Check sheet for the modelled part. Datum: model origin and axes. Units: mm. Coordinates: 2 decimals unless noted, no trailing zeros. Loops run counter-clockwise (first coordinate to the right, second up) from the corner with the lowest first, then second, coordinate; pieces in that order, holes last.
from build123d import *

# Parameters (mm, degrees)
SKETCH1_R           = 1.5
BOSS_EXTRUDE1_DEPTH = 5
SKETCH8_R           = 1.5
CUT_EXTRUDE5_DEPTH  = 10
SKETCH9_R           = 1.5
CUT_EXTRUDE6_DEPTH  = 10


with BuildPart() as part:
    # Sketch1 → Boss-Extrude1 (new body)
    with BuildSketch(Plane(origin=(0, 0, 0), x_dir=(1, 0, 0), z_dir=(0, 1, 0))):
        with BuildLine():
            Line((100, -40), (100, 10))
            Line((100, 10), (40, 150))
            Line((40, 150), (-40, 150))
            Line((-40, 150), (-100, 10))
            Line((-100, 10), (-100, -40))
            ThreePointArc((-100, -40), (-97.071067812, -47.071067812), (-90, -50))
            Line((-90, -50), (-70, -50))
            Line((-70, -50), (-70, -60))
            Line((-70, -60), (-70, -110))
            ThreePointArc((-70, -110), (-67.071067812, -117.071067812), (-60, -120))
            Line((-60, -120), (60, -120))
            ThreePointArc((60, -120), (67.071067812, -117.071067812), (70, -110))
            Line((70, -110), (70, -60))
            Line((70, -60), (70, -50))
            Line((70, -50), (90, -50))
            ThreePointArc((90, -50), (97.071067812, -47.071067812), (100, -40))
        make_face()
        with Locations((-60, -60)):
            Circle(SKETCH1_R, mode=Mode.SUBTRACT)
        with Locations((60, -60)):
            Circle(SKETCH1_R, mode=Mode.SUBTRACT)
    extrude(amount=BOSS_EXTRUDE1_DEPTH)

    # Sketch8 → Cut-Extrude5 (cut)
    with BuildSketch(Plane(origin=(0, 5, 0), x_dir=(1, 0, 0), z_dir=(0, 1, 0))):
        with Locations((-90, 10)):
            Circle(SKETCH8_R)
        with Locations((-32, 140)):
            Circle(SKETCH8_R)
        with Locations((90, 10)):
            Circle(SKETCH8_R)
        with Locations((32, 140)):
            Circle(SKETCH8_R)
    extrude(amount=-CUT_EXTRUDE5_DEPTH, mode=Mode.SUBTRACT)

    # Sketch9 → Cut-Extrude6 (cut)
    with BuildSketch(Plane(origin=(0, 5, 0), x_dir=(1, 0, 0), z_dir=(0, 1, 0))):
        with Locations((47.5, -50)):
            Circle(SKETCH9_R)
        with Locations((32.5, -50)):
            Circle(SKETCH9_R)
        with Locations((32.5, -92)):
            Circle(SKETCH9_R)
        with Locations((-32.5, -50)):
            Circle(SKETCH9_R)
        with Locations((-32.5, -92)):
            Circle(SKETCH9_R)
        with Locations((-47.5, -50)):
            Circle(SKETCH9_R)
    extrude(amount=-CUT_EXTRUDE6_DEPTH, mode=Mode.SUBTRACT)


solid = part.part
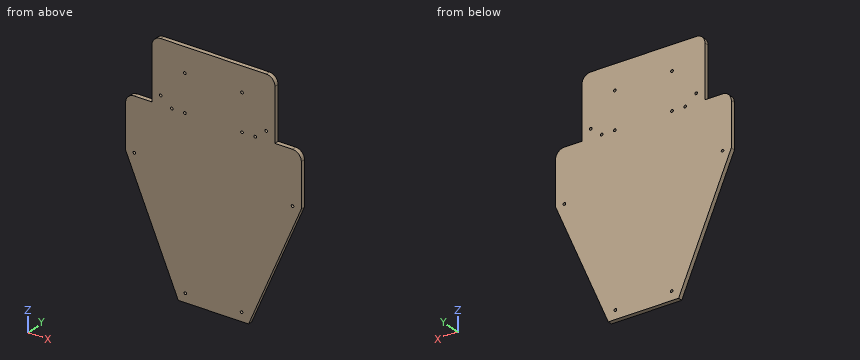
(1) Gauge pin test, flat ends, axial feed: P1, Ø2.5, axis at x = 60, z = 60, coming from the +Y side; P2, Ø2, axis at y = 3, z = 42, coming from the -X side; P3, Ø3, axis at x = -66, y = 3.5, coming from the +Z side; P4, Ø1, axis at x = 78, y = 3.5, coming from the -Z side. Record the tip position at first contact, or that the pin passes through.
(2) Section check B-B, the plane z = 67. Enter the section's corners in (x, y).
(3) Scan lines: line 1 along X through (y, z) = (4.65, 92); line 2 along X through (y, z) = (1.6, -10); line 3 along Z through (x, y) = (32.5, 3.85). Record each from-to range of solid material in increasing order.
(4) Section check A-A, the plane y = 2.9. Count the separate pieces of the cut face and the enclosed holes in it, plus the area to 3 significant figures.
(5) Section check C-C, the plane x = 54.5. Enter the section's corners in (y, z), plus the area to 3 significant figures.
Determined:
1. P1: passes through
1. P2: stops at x = -99.95
1. P3: stops at z = 118.93
1. P4: stops at z = -62.5
2. outline: (-70, 0) - (70, 0) - (70, 5) - (-70, 5) - close
3. line 1: x = -70 to -34, -31 to 31, 34 to 70
3. line 2: x = -100 to -91.5, -88.5 to 88.5, 91.5 to 100
3. line 3: z = -150 to -141.41, -138.59 to 48.5, 51.5 to 90.5, 93.5 to 120
4. separate pieces: 1
4. enclosed holes: 12
4. area: 41,200 mm2
5. outline: (0, -116.17) - (5, -116.17) - (5, 120) - (0, 120) - close
5. area: 1,180 mm2
